For this review, take the finished solid that the model builds, in its own axes (mm). A direction names the side the tool comes from. Give positions to 0.01 mm unless a question says otherwise; leave off trailing zeros. Order: outer loops, then holes, each group sorted by start corner. A loop starts at its lowest first (then second) coordinate and runs counter-clockwise, first axis right, second up.
from build123d import *

# Parameters (mm, degrees)
BOSS_EXTRUDE1_DEPTH = 12.7
SKETCH2_R           = 6.35
CUT_EXTRUDE1_DEPTH  = 128
FILLET1_R           = 1.27
HOLE1_D             = 7.94512
HOLE1_DEPTH         = 68.2625
HOLE1_TIP           = 2.386954861


with BuildPart() as part:
    # Sketch1 → Boss-Extrude1 (new body, symmetric)
    with BuildSketch(Plane.XY):
        Polygon((4.7625, 0), (-4.7625, 0), (-4.7625, 38.1), (-63.5, 38.1), (-63.5, 171.45), (-49.2125, 171.45), (-49.2125, 158.75), (-50.8, 158.75), (-50.8, 47.625), (50.8, 47.625), (50.8, 158.75), (49.2125, 158.75), (49.2125, 171.45), (63.5, 171.45), (63.5, 38.1), (4.7625, 38.1), align=None)
    extrude(amount=BOSS_EXTRUDE1_DEPTH, both=True)

    # Sketch2 → Cut-Extrude1 (cut, through all)
    with BuildSketch(Plane.ZY.offset(63.5)):
        with Locations((0, 76.2)):
            Circle(SKETCH2_R)
        with Locations((0, 139.7)):
            Circle(SKETCH2_R)
    extrude(amount=-CUT_EXTRUDE1_DEPTH, mode=Mode.SUBTRACT)

    # Fillet1
    fillet1_edges = [part.edges().sort_by_distance(p)[0] for p in [
        (4.7625, 0, 0),
        (-4.7625, 0, 0),
        (-50.8, 158.75, 0),
        (-50.8, 47.625, 0),
        (50.8, 47.625, 0),
        (50.8, 158.75, 0),
    ]]
    fillet(fillet1_edges, radius=FILLET1_R)

    # Hole1
    with Locations(Plane(origin=(4.7625, 0, 0), x_dir=(0, 0, 1), z_dir=(1, 0, 0))):
        with Locations((0, -25.4), (0, -10.16)):
            Hole(HOLE1_D / 2, depth=HOLE1_DEPTH)
            with Locations((0, 0, -(HOLE1_DEPTH + HOLE1_TIP / 2))):  # 118° drill point
                Cone(0, HOLE1_D / 2, HOLE1_TIP, mode=Mode.SUBTRACT)


solid = part.part
1) We need section D-D on x = 9.5. Give the boundary of the cut face in (y, z) (3 decimals).
Answer sheet:
outline: (38.1, -12.7) - (47.625, -12.7) - (47.625, 12.7) - (38.1, 12.7) - close
2) We need section A-A on y = 88. Give the boundary of the cut face in (x, z).
Answer sheet:
outline: (-63.5, -12.7) - (-50.8, -12.7) - (-50.8, 12.7) - (-63.5, 12.7) - close; (50.8, -12.7) - (63.5, -12.7) - (63.5, 12.7) - (50.8, 12.7) - close
3) Tool access review of faces 4 (the face through (50.8, 102, 0)), 5 (the face through (4.762, 20, 0)), 6 (the face through (-34, 38.1, 0)), 7 (the face through (49.212, 165, 0)): name each direction out of +Z, -Z, +X, -X, +Y, -Y from which nothing blocks a thin tool from reaching the whole face with its end or side.
Answer sheet:
face 4: +Z, -Z
face 5: +Z, -Z, +X, -Y
face 6: +Z, -Z, -X, -Y
face 7: +Z, -Z, +Y
4) We need section C-C on z = 0. Count the separate pieces of the cut face and the enclosed holes in it, then the cut area to 3 significant figures.
Answer sheet:
separate pieces: 7
enclosed holes: 0
area: 3,960 mm2
5) To check wall thickness, follow line 1 (Y direction, x = -59.75, z = 0); line 2 (Y direction, x = 1.5, z = 0) (3 decimals); line 3 (X direction, y = 129, z = 8.5). State the ranges of each line that lie inside material, in increasing order.
Answer sheet:
line 1: y = 38.1 to 69.85, 82.55 to 133.35, 146.05 to 171.45
line 2: y = 0 to 6.187, 14.133 to 21.427, 29.373 to 47.625
line 3: x = -63.5 to -50.8, 50.8 to 63.5
6) Draft analysis for pull direction Y (two halves, no side actions). For faces 1 (the face through (-57.24, 70, -1.38)), 2 (the face through (0, 0, 0)), 3 (the face through (56, 171.45, 0)), state which applies: +Y half, -Y half, draft (parallel to the pull), parting line (faces both ways), or undercut.
Answer sheet:
face 1: undercut
face 2: -Y half
face 3: +Y half
7) Clearance check with flat-ended pins moving along their axes: pin 1 (2 mm diameter, centred on x = 13.5, z = 6, fed in from -Y); pin 2 (12.5 mm diameter, centred on y = 11, z = 1, fed in from +X); pin 3 (11.5 mm diameter, centred on y = 139.7, z = 0, fed in from -X); pin 4 (3 mm diameter, centred on x = -34.5, z = -1, fed in from +Y) (3 decimals). State where each tip first meets the part, or that it passes through.
Answer sheet:
pin 1: stops at y = 38.1
pin 2: stops at x = 4.76
pin 3: passes through
pin 4: stops at y = 47.625
